Source: three-view drawing plus pictorial views. Frame: mm from the lowest corner of the part. A direction names the side the tool comes from. Round coordinates to 2 decimals unless told otherwise and drop trailing zeros. Write each loop counter-clockwise with the first axis right and the second up, starting at its lowest first coordinate (ties: lowest second). Pieces come first, ordered by that corner, then holes. Notation, with made-up numbers: (-13.75, -6.5) -> (9.25, -6.5) arc R26 ccw to (9.25, 22.5) -> close; hole circle Ø1 at (2.5, 77). An arc over 180 degrees is marked (long way). Put each result on its own line as item: value.
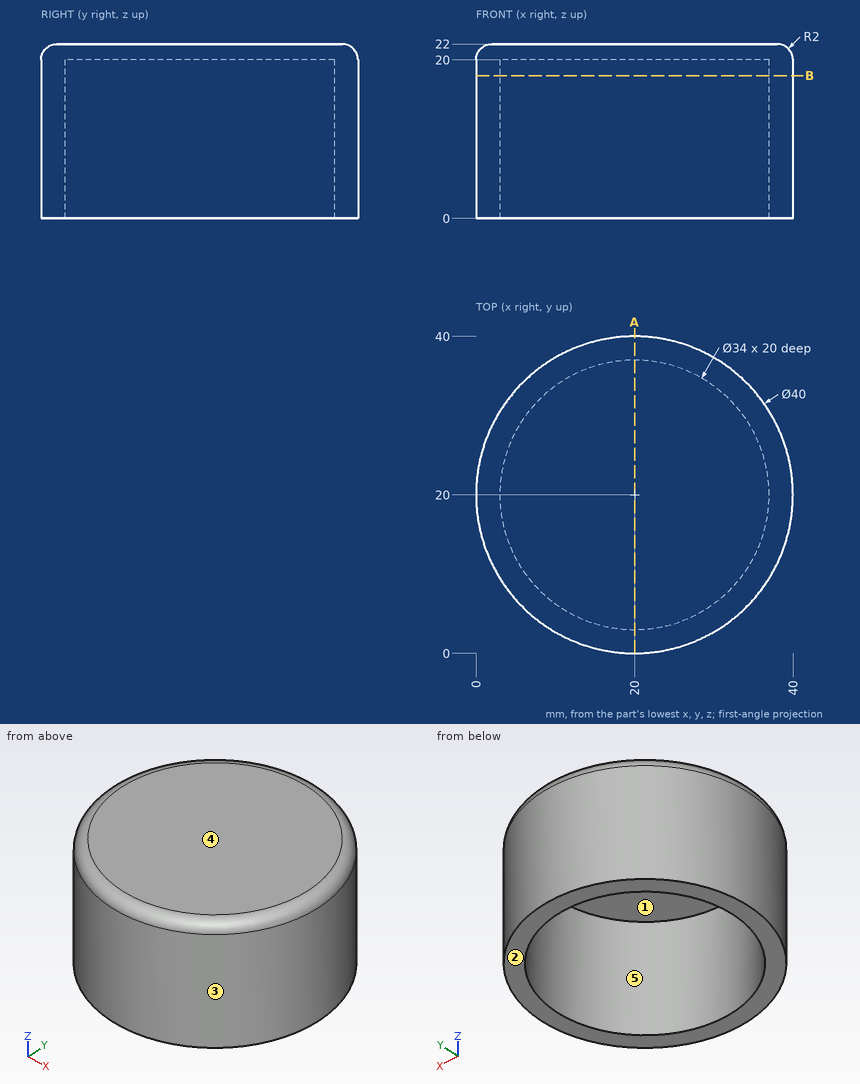
Q1. Cut plane B-B on z = 18. Output: boundary loops of the cut face in (x, y).
Ans:
outline: circle Ø40 at (20, 20); hole circle Ø34 at (20, 20)
Q2. Cut plane A-A on x = 20. Output: boundary loops of the cut face in (y, z), and give its area (3 significant figures).
Ans:
outline: (0, 0) -> (3, 0) -> (3, 20) -> (37, 20) -> (37, 0) -> (40, 0) -> (40, 20) arc R2 ccw to (38, 22) -> (2, 22) arc R2 ccw to (0, 20) -> close
area: 198 mm^2
Q3. Reachability of the marked faces 4 and 5 from +Z, -Z, +X, -X, +Y, -Y: full face, straight path, thin tool, end or side. Return the list, or none.
Ans:
face 4: +Z, +X, -X, +Y, -Y
face 5: -Z
Q4. Pin query (flat end, axial travel): pin 1 (1.5 mm diameter, centred on y = 6, z = 12.5, fed in from -X); pin 2 (12 mm diameter, centred on x = 31.5, z = 6.5, fed in from +Y); pin 3 (6 mm diameter, centred on y = 6.5, z = 10, fed in from -X). Return the tip coordinate at first contact, or that it passes through.
Ans:
pin 1: stops at x = 5.02
pin 2: stops at y = 39.23
pin 3: stops at x = 2.98
Q5. Draft query along Y for the marked faces 1, 2 and 3. Return one class per face: +Y half, -Y half, draft (parallel to the pull), parting line (faces both ways), or undercut.
Ans:
face 1: undercut
face 2: draft
face 3: parting line
Q6. Material intervals for line 1 (Y direction, x = 20, z = 16.25); line 2 (X direction, y = 26.5, z = 2.25); line 3 (Y direction, x = 8, z = 10.5), sorted ascending. Write a range as [from, to].
Ans:
line 1: y = [0, 3], [37, 40]
line 2: x = [1.09, 4.29], [35.71, 38.91]
line 3: y = [4, 7.96], [32.04, 36]
